from build123d import *

# Parameters (mm, degrees)
BOSS_EXTRUDE1_DEPTH = 80
SKETCH2_R           = 2
CUT_EXTRUDE1_DEPTH  = 4
CUT_EXTRUDE2_START  = -4
SKETCH3_R           = 2
CUT_EXTRUDE2_DEPTH  = 4


with BuildPart() as part:
    # Sketch1 → Boss-Extrude1 (new body)
    with BuildSketch(Plane.XY):
        with BuildLine():
            Line((-15, 0), (15, 0))
            Line((15, 0), (15, 2.5))
            Line((15, 2.5), (35, 2.5))
            Line((35, 2.5), (35, -10))
            Line((35, -10), (12.8, -10))
            Line((12.8, -10), (12.8, -12))
            ThreePointArc((12.8, -12), (13.385786438, -13.414213562), (14.8, -14))
            Line((14.8, -14), (37, -14))
            ThreePointArc((37, -14), (38.414213562, -13.414213562), (39, -12))
            Line((39, -12), (39, 4.5))
            ThreePointArc((39, 4.5), (38.414213562, 5.914213562), (37, 6.5))
            Line((37, 6.5), (15, 6.5))
            Line((15, 6.5), (-15, 6.5))
            Line((-15, 6.5), (-37, 6.5))
            ThreePointArc((-37, 6.5), (-38.414213562, 5.914213562), (-39, 4.5))
            Line((-39, 4.5), (-39, -12))
            ThreePointArc((-39, -12), (-38.414213562, -13.414213562), (-37, -14))
            Line((-37, -14), (-14.8, -14))
            ThreePointArc((-14.8, -14), (-13.385786438, -13.414213562), (-12.8, -12))
            Line((-12.8, -12), (-12.8, -10))
            Line((-12.8, -10), (-35, -10))
            Line((-35, -10), (-35, 2.5))
            Line((-35, 2.5), (-15, 2.5))
            Line((-15, 2.5), (-15, 0))
        make_face()
    extrude(amount=BOSS_EXTRUDE1_DEPTH)

    # Sketch2 → Cut-Extrude1 (cut)
    with BuildSketch(Plane.XZ.offset(-2.5)):
        with Locations((-28.8, 60)):
            Circle(SKETCH2_R)
        with Locations((28.8, 60)):
            Circle(SKETCH2_R)
        with Locations((28.8, 40)):
            Circle(SKETCH2_R)
        with Locations((28.8, 20)):
            Circle(SKETCH2_R)
        with Locations((-28.8, 40)):
            Circle(SKETCH2_R)
        with Locations((-28.8, 20)):
            Circle(SKETCH2_R)
    extrude(amount=-CUT_EXTRUDE1_DEPTH, mode=Mode.SUBTRACT)

    # Sketch3 → Cut-Extrude2 (cut)
    with BuildSketch(Plane(origin=(0, -10, 0), x_dir=(1, 0, 0), z_dir=(0, 1, 0)).offset(CUT_EXTRUDE2_START)):
        with Locations((28.8, -40)):
            Circle(SKETCH3_R)
    extrude(amount=CUT_EXTRUDE2_DEPTH, mode=Mode.SUBTRACT)


solid = part.part
Part model, mm, in its own coordinate system. A direction names the side the tool comes from. Coordinates: 2 decimals unless noted, no trailing zeros. Write each loop counter-clockwise with the first axis right and the second up, starting at its lowest first coordinate (ties: lowest second). Pieces come first, ordered by that corner, then holes. Notation, with made-up numbers: M 59,76 L 106,76 A15 ccw 106,90 Z; hole C -9,-29 d11. An arc over 180 degrees is marked long. Return JSON: item names as keys, results as strings.
1. Pull direction X, two halves, no side cores. Call faces 4 (the face through (-9, 1, 0)), 5 (the face through (38.4, -13.43, 39.44)), 6 (the face through (27.326, 4.472, 21.352)), 7 (the face through (-39, -4, 39)): pulls with the +X half, pulls with the -X half, needs draft (parallel to the pull), parting line crosses it, or undercut.
Determined:
{"face 4": "needs draft", "face 5": "pulls with the +X half", "face 6": "undercut", "face 7": "pulls with the -X half"}
2. 3-axis set-ups, long thin cutter, end or side, ignore diameter. For faces 1 (the face through (35, -4, 39)), 2 (the face through (-12.8, -11, 39)), 3 (the face through (-27.725, 4.472, 61.686)): which of +Z, -Z, +X, -X, +Y, -Y reach the whole face in a straight line?
Determined:
{"face 1": "+Z, -Z", "face 2": "+Z, -Z, -Y", "face 3": "+Y"}
3. Flat gauge pins, fed straight in: pin 1 Ø4.5 at (x, z) = (-28.8, 40) entering from +Y; pin 2 Ø3.5 at (x, z) = (28.8, 40) entering from +Y; pin 3 Ø15 at (x, z) = (-1.5, 45) entering from -Y. Where does each tip first touch, or does it go through?
Determined:
{"pin 1": "y = 6.5", "pin 2": "through", "pin 3": "y = 0"}
4. Probe L1, parallel to X at y = -12.05, z = 40; L2, parallel to Z at x = -28.8, y = 5.55; L3, parallel to Y at x = -27, z = 71.5. List the from-to ranges inside material, lowest first.
Determined:
{"L1": "-39 to -12.8, 12.8 to 26.8, 30.8 to 39", "L2": "0 to 18, 22 to 38, 42 to 58, 62 to 80", "L3": "-14 to -10, 2.5 to 6.5"}
5. Saw through at B-B, the plane z = 60. Count the separate pieces of the cut face and the enclosed holes in it, then the cut area to 3 significant figures.
Determined:
{"separate pieces": "3", "enclosed holes": "0", "area": "659 mm²"}
6. Saw through at C-C, the plane x = 28.8. Write the cut outline in (y, z), then the cut area to 3 significant figures.
Determined:
{"outline": "M -14,0 L -10,0 L -10,38 L -14,38 Z; M -14,42 L -10,42 L -10,80 L -14,80 Z; M 2.5,0 L 6.5,0 L 6.5,18 L 2.5,18 Z; M 2.5,22 L 6.5,22 L 6.5,38 L 2.5,38 Z; M 2.5,42 L 6.5,42 L 6.5,58 L 2.5,58 Z; M 2.5,62 L 6.5,62 L 6.5,80 L 2.5,80 Z", "area": "576 mm²"}
7. Saw through at A-A, the plane y = 1.25. Write the cut outline in (x, z), then the cut area to 3 significant figures.
Determined:
{"outline": "M -39,0 L -35,0 L -35,80 L -39,80 Z; M -15,0 L 15,0 L 15,80 L -15,80 Z; M 35,0 L 39,0 L 39,80 L 35,80 Z", "area": "3,040 mm²"}
